```python
from build123d import *

# Parameters (mm, degrees)
SKETCH_1_R      = 85
SKETCH_1_R_2    = 15
EXTRUDE_1_DEPTH = 1
SKETCH_1_3_R    = 15
SKETCH_1_3_R_2  = 12.5
EXTRUDE_2_DEPTH = 81
SKETCH_1_4_R    = 12.5
EXTRUDE_3_DEPTH = 120


with BuildPart() as part:
    # Sketch 1 → Extrude 1 (new body)
    with BuildSketch(Plane.XY):
        Circle(SKETCH_1_R)
        Circle(SKETCH_1_R_2, mode=Mode.SUBTRACT)
    extrude(amount=EXTRUDE_1_DEPTH)

    # Sketch 1_3 → Extrude 2 (add)
    # profile 1 of 2: a face of its own
    with BuildSketch(Plane.XY):
        Circle(SKETCH_1_3_R)
        Circle(SKETCH_1_3_R_2, mode=Mode.SUBTRACT)
    # profile 2 of 2: a face of its own
    with BuildSketch(Plane.XY):
        Circle(SKETCH_1_3_R_2)
    extrude(amount=EXTRUDE_2_DEPTH)

    # Sketch 1_4 → Extrude 3 (add)
    with BuildSketch(Plane.XY):
        Circle(SKETCH_1_4_R)
    extrude(amount=EXTRUDE_3_DEPTH)


solid = part.part
```
Geometry: final body of the model. Coordinates: model frame, mm. A direction names the side the tool comes from. Coordinates: 2 decimals unless noted, no trailing zeros. Order: outer loops, then holes, each group sorted by start corner. A loop starts at its lowest first (then second) coordinate and runs counter-clockwise, first axis right, second up. Notation, with made-up numbers: (11, 33.25) - (63, 33.25) arc R26 ccw to (63, 67.25) - close; hole circle Ø8 at (43.25, -15). An arc over 180 degrees is marked (long way). Write each question's results on one line, items separated by ' | '.
(1) Set-up query: faces 1 (the face through (11.923, 3.755, 100.227)), 2 (the face through (-67.453, -51.721, 0.493)). Return all of +Z, -Z, +X, -X, +Y, -Y with unobstructed straight access to the full face (end or side cutting, diameter ignored); none if empty.
Values found:
face 1: +Z | face 2: +Z, -Z
(2) Line query: line 1 (Z direction, x = 12, y = -35.5); line 2 (X direction, y = 3.5, z = 60); line 3 (X direction, y = 5.5, z = 30). Output: solid intervals per line, ascending. Write a range as [from, to].
Values found:
line 1: z = [0, 1] | line 2: x = [-14.59, 14.59] | line 3: x = [-13.96, 13.96]
(3) Section query D-D, the plane z = 51. Return the cut outline in (x, y).
Values found:
outline: circle Ø30 at (0, 0)
(4) Section query A-A, the plane x = 0. Return the cut outline in (y, z), plus the area to 4 significant figures.
Values found:
outline: (-85, 0) - (85, 0) - (85, 1) - (15, 1) - (15, 81) - (12.5, 81) - (12.5, 120) - (-12.5, 120) - (-12.5, 81) - (-15, 81) - (-15, 1) - (-85, 1) - close | area: 3,545 mm²
(5) Section query C-C, the plane z = 96. Return the cut outline in (x, y).
Values found:
outline: circle Ø25 at (0, 0)
(6) First-contact query: pin 1 Ø5 at (x, y) = (55, 39.5) entering from +Z; pin 2 Ø1 at (x, z) = (4.5, 43) entering from +Y; pin 3 Ø4 at (y, z) = (5.5, 98.5) entering from -X; pin 4 Ø1.5 at (x, y) = (23, 35) entering from -Z. Flat tips, straight axial feed; report the tip coordinate or a pass-through.
Values found:
pin 1: stops at z = 1 | pin 2: stops at y = 14.46 | pin 3: stops at x = -12 | pin 4: stops at z = 0
